Could you check a few things on this model? Use its own coordinates, in mm. A direction names the side the tool comes from. Coordinates: 2 decimals unless noted, no trailing zeros. Loops run counter-clockwise (first coordinate to the right, second up) from the corner with the lowest first, then second, coordinate; pieces in that order, holes last. Notation, with made-up numbers: (34.25, 16.5) - (38.25, 16.5) arc R16 cw to (38.25, 31.5) - close; hole circle Ø11 at (-12.5, -35.5). An arc over 180 degrees is marked (long way). Put each result on its own line as item: value. Start each with the question number.
Autodesk Inventor part; units mm, degrees
ref_plane "YZ Plane" through (0, 0, 0) normal (1, 0, 0) x (0, 1, 0)
ref_plane "XZ Plane" through (0, 0, 0) normal (0, 1, 0) x (-1, 0, 0)
ref_plane "XY Plane" through (0, 0, 0) normal (0, 0, 1) x (1, 0, 0)
sketch "Skizze3" plane through (0, 0, 0) normal (0, 0, 1) x (1, 0, 0)
  line L0 (-500, 500) -> (500, 500)
  line L1 (500, 500) -> (500, -500)
  line L2 (500, -500) -> (-500, -500)
  line L3 (-500, -500) -> (-500, 500)
  line L4 (-500, -400) -> (500, -400)
  line L5 (-275, 500) -> (275, 500)
  line L6 (275, 500) -> (275, 320)
  line L7 (275, 320) -> (-275, 320)
  line L8 (-275, 320) -> (-275, 500)
  arc A0 (-275, 320) -> (-400, -400) centre (1736.1, -400) ccw
  arc A1 (400, -400) -> (275, 320) centre (-1736.1, -400) ccw
  line L9 (-160, 320) -> (160, 320)
  line L10 (160, 320) -> (160, 360)
  line L11 (160, 360) -> (-160, 360)
  line L12 (-160, 360) -> (-160, 320)
  line L13 (-440, -450) -> (-140, -450)
  line L14 (90, -450) -> (440, -450)
  line L15 (-30, 360) -> (-30, 320)
  arc A2 (-440, -450) -> (-160, 320) centre (-1358.75, 320) ccw
  arc A3 (-140, -450) -> (-30, 320) centre (-2780, 320) ccw
  arc A4 (-30, 320) -> (90, -450) centre (2500.4167, 320) ccw
  arc A5 (160, 320) -> (440, -450) centre (1358.75, 320) ccw
  line L16 (-160, 360) -> (-440, -450) construction
  line L17 (-160, 360) -> (-146.1239, 400.1416) construction
  line L18 (-30, 360) -> (-146.1239, 400.1416) construction
  line L19 (-30, 360) -> (121.8543, 307.5071) construction
  line L20 (-440, -450) -> (-172.0218, -542.6344) construction
  line L21 (-140, -450) -> (-172.0218, -542.6344) construction
  line L22 (-140, -450) -> (121.8543, 307.5071) construction
  line L23 (-172.9217, 310.595) -> (139.7195, 418.6685) construction
  line L24 (139.7195, 418.6685) -> (440, -450) construction
  line L25 (440, -450) -> (127.3587, -558.0735) construction
  line L26 (127.3587, -558.0735) -> (-172.9217, 310.595) construction
  point P0 (0, 0)
  point P1 (-500, 0)
  point P2 (0, 500)
  point P3 (0, 320)
  point P4 (0, 360)
  dimension "d4" = 1000
  dimension "d5" = 1000
  dimension "d6" = 100
  dimension "d7" = 550
  dimension "d8" = 180
  dimension "d9" = 100
  dimension "d10" = 100
  dimension "d11" = 320
  dimension "d12" = 300
  dimension "d13" = 350
  dimension "d14" = 230
  dimension "d15" = 60
  dimension "d16" = -60
  dimension "d17" = 130
  dimension "d18" = 190
  dimension "d19" = 50
  dimension "d21" = 283.5374
  dimension "d22" = 40
  dimension "d23" = 140
  dimension "d24" = 899.502
  dimension "d25" = 919.1046
  dimension "d26" = 330.7937
extrude "Extrusion6" add sketch "Skizze3" along normal blind 40 contours A2 A0 L4 | L4 A3 L13 A2 | L12 L11 L15 L7 | L7 A3 L4 A0 A2
equation "\"d9\" = d6"
equation "\"d10\" = d6"
properties part number "UA-072-PlatteLinks"
(1) I want a section at C-C on x = -361. List the corners of the cut face in (y, z) for me.
(2) I want a section at A-A on z = 33. List the corners of the cut face in (x, y) for me.
(3) For pin 1 Ø1.5 at (y, z) = (-208.5, 17) entering from +X; pin 2 Ø5 at (x, y) = (-173, 167.5) entering from +Z; pin 3 Ø12 at (x, z) = (-371.5, 14) entering from +Y; pin 4 Ø3 at (y, z) = (150, 34.5) entering from -X, each with a flat end and sliding along its axis, tell me the tip position at first contact or that it passes through.
(4) I want a section at B-B on y = -311. List the corners of the cut face in (x, z) for me, and give its area (3 significant figures).
(5) I need wall thicknesses on L1, parallel to X at y = 319, z = 22; L2, parallel to X at y = -267, z = 13.5; L3, parallel to Y at x = -314, z = 6. Which ranges of each line are inside material? Lowest first, please. Write a range as [from, to].
(6) Which directions (+Z, -Z, +X, -X, +Y, -Y) give clear straight access to the entire face, cutting with the end or side of a thin tool? Please do faces 1 (the flat face through (-147, -129, 0)), 2 (the flat face through (-160, 340, 20)).
Answer sheet:
1. outline: (-450, 0) - (-344.45, 0) - (-344.45, 40) - (-450, 40) - close
2. outline: (-440, -450) - (-140, -450) arc R2750 ccw to (-30, 320) - (-30, 360) - (-160, 360) - (-160, 320) arc R1198.75 cw to start
3. pin 1: stops at x = -81.12
3. pin 2: passes through
3. pin 3: stops at y = -351.16
3. pin 4: stops at x = -172.33
4. outline: (-339.51, 0) - (-103.37, 0) - (-103.37, 40) - (-339.51, 40) - close
4. area: 9,450 mm^2
5. L1: x = [-160, -30]
5. L2: x = [-313.56, -93.38]
5. L3: y = [-450, -267.79]
6. face 1: -Z, +X, -X, +Y, -Y
6. face 2: +Z, -Z, -X, +Y
